Autodesk Inventor part; units mm, degrees
ref_plane "YZ Plane" through (0, 0, 0) normal (1, 0, 0) x (0, 1, 0)
ref_plane "XZ Plane" through (0, 0, 0) normal (0, 1, 0) x (-1, 0, 0)
ref_plane "XY Plane" through (0, 0, 0) normal (0, 0, 1) x (1, 0, 0)
sketch "스케치1" plane through (0, 0, 0) normal (0, 0, 1) x (1, 0, 0)
  line L0 (0, 0) -> (4, 0)
  line L1 (4, 0) -> (4, 12)
  line L2 (4, 12) -> (0, 12)
  line L3 (0, 12) -> (0, 0)
  dimension "d0" = 4
  dimension "d1" = 12
extrude "돌출1" add sketch "스케치1" along normal blind 3
sketch "스케치2" plane through (0, 0, 3) normal (0, 0, 1) x (1, 0, 0)
  line L0 (4, 12) -> (0, 12) construction
  line L1 (2, 12) -> (2, 0) construction
  line L2 (0, 0) -> (4, 0) construction
  line L3 (4, 0) -> (4, 12)
  line L4 (0, 12) -> (0, 0)
  point P0 (2, 7.7)
  point P1 (2, 4.3)
  point P2 (2, 1.3)
  point P3 (2, 10.7)
  dimension "d9" = 4.3
  dimension "d45" = 1.3
  dimension "d51" = 3.4
  dimension "d52" = 3
  dimension "d55" = 1.3
hole "구멍2" at (2, 4.3, 3) direction (0, 0, -1) diameter 1.6 end through all
hole "구멍3" at (2, 1.3, 3) at (2, 10.7, 3) direction (0, 0, -1) diameter 1 end through all
sketch "스케치5" plane through (0, 0, 0) normal (-1, 0, 0) x (0, 0, 1)
  line L0 (0, 12) -> (0, 0)
  line L1 (0, 0) -> (3, 0)
  line L2 (3, 12) -> (3, 0)
  line L3 (0, 12) -> (3, 12)
  line L4 (-1, 12) -> (4.5, 12)
  line L5 (4.5, 12) -> (4.5, 0)
  line L6 (4.5, 0) -> (-1, 0)
  line L7 (-1, 0) -> (-1, 12)
  line L8 (0, 0) -> (3, 0)
  dimension "d62" = 4.5
  dimension "d71" = 1
extrude "돌출5" add sketch "스케치5" along normal blind 2
sketch "스케치6" plane through (-2, 0, 0) normal (-1, 0, 0) x (0, 0, 1)
  line L0 (4.5, 0) -> (4.5, 12)
  line L1 (-1, 12) -> (-1, 0)
  line L2 (-1, 0) -> (4.5, 0)
  line L3 (4.5, 0) -> (4.5, 12)
  line L4 (4.5, 12) -> (-1, 12)
  line L5 (-1, 12) -> (-1, 10.7)
  line L6 (-1, 10.7) -> (4.5, 10.7)
  line L7 (4.5, 10.7) -> (4.5, 12)
  line L8 (-1, 12) -> (-1, 0)
  line L9 (-1, 0) -> (4.5, 0)
  line L10 (4.5, 0) -> (4.5, 1.3)
  line L11 (4.5, 1.3) -> (-1, 1.3)
  line L12 (-1, 1.3) -> (-1, 0)
  line L13 (-1, 12) -> (-1, 0)
  line L14 (-1, 9.2) -> (0.5, 10.7)
  line L15 (-1, 2.8) -> (0.5, 1.3)
  line L16 (4.5, 12) -> (-1, 12)
  point P0 (-1, 1.3)
  point P1 (4.5, 10.7)
  point P2 (-1, 12)
  dimension "d72" = 9.4
  dimension "d74" = 1.3
  dimension "d78" = 1.5
  dimension "d79" = 45
  dimension "d80" = 45
extrude "돌출6" add sketch "스케치6" along normal blind 1 contours L2 L1 L11 L0 | L6 L1 L4 L0 | L11 L1 L15 | L14 L1 L6
chamfer "모따기2" distance 0.5 angle 45 1 edges at (0, 6, 0)
sketch "스케치7" plane through (-2, 0, 0) normal (-1, 0, 0) x (0, 0, 1)
  line L0 (-1, 2.8) -> (0.5, 1.3)
  line L1 (0.5, 1.3) -> (4.5, 1.3)
  line L2 (4.5, 1.3) -> (4.5, 10.7)
  line L3 (4.5, 10.7) -> (0.5, 10.7)
  line L4 (0.5, 10.7) -> (-1, 9.2)
  line L5 (-1, 9.2) -> (-1, 2.8)
extrude "돌출7" cut sketch "스케치7" against normal blind 0.5
sketch "스케치8" plane through (-3, 1.3, 4.5) normal (0, 1, 0) x (1, 0, 0)
  line L0 (1.5, 4) -> (1.5, 0)
  arc A0 (1.5, 1) -> (1.5, 4.5) centre (-4.2391, 2.75) ccw
  line L1 (7, 4.5) -> (3.5, 4.5)
  line L2 (3, 5) -> (3.5, 4.5)
  line L3 (3, 5.5) -> (0, 5.5)
  line L4 (3, 0) -> (0, 0)
  line L5 (7, 1.5) -> (3, 1.5)
  line L6 (7, 4.5) -> (7, 1.5)
  line L7 (1.5, 1) -> (1.5, 4.5)
  line L8 (1.5, 4) -> (1.5, 5.5)
  line L9 (0, 0) -> (0, 5.5)
  line L10 (3, 5) -> (3, 5.5)
  line L11 (3, 0) -> (3, 1.5)
  point P0 (3, 4.5)
  point P1 (1.5, 4)
  dimension "d84" = 6
extrude "돌출8" cut sketch "스케치8" along normal up to surface (9.4 mm away) contours L7 A0 L0
chamfer "모따기3" distance 0.5 distance2 1.5 1 edges at (0, 6, 3) measured on face at (3.5981, 5.4655, 3)
sketch "스케치9" plane through (-3, 0, 0) normal (-1, 0, 0) x (0, 0, 1)
  line L0 (-1, 12) -> (-1, 9.2)
  line L1 (-1, 9.2) -> (0.5, 10.7)
  line L2 (0.5, 10.7) -> (4.5, 10.7)
  line L3 (4.5, 0) -> (4.5, 1.3)
  line L4 (2, 12) -> (2, 10.7)
  line L5 (0.5, 10.7) -> (4.5, 10.7)
  line L6 (-1, 0) -> (4.5, 0)
  line L7 (4.5, 1.3) -> (0.5, 1.3)
  line L8 (0.5, 1.3) -> (-1, 2.8)
  line L9 (-1, 2.8) -> (-1, 0)
  line L10 (4.5, 12) -> (-1, 12)
  line L11 (4.5, 10.7) -> (4.5, 12)
  point P0 (0, 0)
  dimension "d91" = 2.5
extrude "돌출9" cut sketch "스케치9" against normal up to surface (1.5 mm away) contours L10 L11 L2 L4
equation "\"d80\" = d79"
equation "\"G23_M\" = 0.67"
equation "\"G23_F\" = 0.65"
properties part number "Top" material "유리"
Work out the finished part from the listing and answer in its coordinate system (mm). A direction names the side the tool comes from. Coordinates: 2 decimals unless noted, no trailing zeros. Loops run counter-clockwise (first coordinate to the right, second up) from the corner with the lowest first, then second, coordinate; pieces in that order, holes last. Notation, with made-up numbers: (84.25, 14.25) -> (117.25, 14.25) arc R28 cw to (117.25, 45.25) -> close; hole circle Ø5 at (66, 43). An arc over 180 degrees is marked (long way). Answer as CSV lines item,"result".
1) Straight lines are drawn through the part: probe 1 along Y at (x, z) = (2, 1.7); probe 2 along X at (y, z) = (4.3, 1.75); probe 3 along Y at (x, z) = (-2.5, 1.7). For each, find the intervals that lie inside material, in ascending order.
A:
probe 1,"y = 0 to 0.8, 1.8 to 3.5, 5.1 to 10.2, 11.2 to 12"
probe 2,"x = -1.24 to 1.2, 2.8 to 4"
probe 3,"y = 0 to 1.3, 10.7 to 12"
2) The part is cut by section C-C (z = 1). Give the vertices of the cut face in (x, y), and give its area (3 significant figures).
A:
outline,"(-3, 0) -> (4, 0) -> (4, 12) -> (-3, 12) -> (-3, 10.7) -> (-1.29, 10.7) -> (-1.29, 1.3) -> (-3, 1.3) -> close; hole circle Ø1.6 at (2, 4.3); hole circle Ø1 at (2, 1.3); hole circle Ø1 at (2, 10.7)"
area,"64.3 mm²"
3) The part is cut by section B-B (x = 2). Give the vertices of the cut face in (y, z), and give its area (3 significant figures).
A:
outline,"(0, 0) -> (0.8, 0) -> (0.8, 3) -> (0, 3) -> close; (1.8, 0) -> (3.5, 0) -> (3.5, 3) -> (1.8, 3) -> close; (5.1, 0) -> (10.2, 0) -> (10.2, 3) -> (5.1, 3) -> close; (11.2, 0) -> (12, 0) -> (12, 3) -> (11.2, 3) -> close"
area,"25.2 mm²"
4) Flat-ended cylindrical pins translate along their axes: pin 1 (1 mm diameter, centred on x = -2.5, y = 11, fed in from +Z); pin 2 (2 mm diameter, centred on y = 7.5, z = 3, fed in from -X); pin 3 (4 mm diameter, centred on x = 3, y = 5, fed in from +Z). Find the tip coordinate at first contact, or state that the pin passes through.
A:
pin 1,"stops at z = 2"
pin 2,"stops at x = -1.5"
pin 3,"stops at z = 3"
5) For a pull along Z with two mould halves and no side action, classify faces 5 (the face through (1.504, 1.365, 1.479)), 6 (the face through (-2.3, 2.1, -0.3)), 7 (the face through (-1.24, 5.93, 1.73)), 8 (the face through (2, 6, 0)) as released by +Z, released by -Z, zero draft, split by the parting line, or undercut.
A:
face 5,"zero draft"
face 6,"released by +Z"
face 7,"undercut"
face 8,"released by -Z"
6) For faces 1 (the face through (-1.5, 7, 4)), 2 (the face through (2, 6, 3)), 3 (the face through (-2.2, 9.9, -0.3)), 4 (the face through (4, 6, 1)), determine the directions among +Z, -Z, +X, -X, +Y, -Y from which every point of the face is accessible in a straight line to the end or side of a thin tool.
A:
face 1,"+Z, -X, +Y"
face 2,"+Z, +X, +Y, -Y"
face 3,"+Z, -X"
face 4,"+Z, -Z, +X, +Y, -Y"
